```python
from build123d import *

# Parameters (mm, degrees)
SKETCH1_W                      = 116.84
SKETCH1_H                      = 76.2
EXTRUDE1_DEPTH                 = 6.35
F_1_4_CLEARANCE_HOLE1_D        = 6.7564
MIRROR2_COPY_1_D               = 6.7564
F_1_2_0_5_DIAMETER_HOLE1_D     = 12.7
F_1_2_0_5_DIAMETER_HOLE1_DEPTH = 17.78
F_1_2_0_5_DIAMETER_HOLE1_TIP   = 3.815464931


with BuildPart() as part:
    # Sketch1 → Extrude1 (new body)
    with BuildSketch(Plane.XY):
        Rectangle(SKETCH1_W, SKETCH1_H)
    extrude(amount=EXTRUDE1_DEPTH)

    # 1/4 Clearance Hole1 (through all)
    with Locations(Plane(origin=(-52.07, 31.75, 6.35), x_dir=(1, 0, 0), z_dir=(0, 0, 1))):
        with Locations((0, 0)):
            f_1_4_clearance_hole1 = Hole(F_1_4_CLEARANCE_HOLE1_D / 2)

    # Mirror1: 1/4 Clearance Hole1 across plane
    add(f_1_4_clearance_hole1.mirror(Plane.ZX), mode=Mode.SUBTRACT)

    # Mirror2: 1/4 Clearance Hole1 across plane
    add(f_1_4_clearance_hole1.mirror(Plane(origin=(0, 0, 0), x_dir=(0, 0, 1), z_dir=(1, 0, 0))), mode=Mode.SUBTRACT)

    # Mirror2 copy 1 (through all)
    with Locations(Plane(origin=(52.07, -31.75, 6.35), x_dir=(-1, 0, 0), z_dir=(0, 0, 1))):
        with Locations((0, 0)):
            Hole(MIRROR2_COPY_1_D / 2)

    # 1/2 (0.5) Diameter Hole1
    with Locations(Plane(origin=(-26.9875, 26.9875, 6.35), x_dir=(1, 0, 0), z_dir=(0, 0, 1))):
        with Locations((0, 0), (53.975, 0), (53.975, -53.975), (0, -53.975)):
            Hole(F_1_2_0_5_DIAMETER_HOLE1_D / 2, depth=F_1_2_0_5_DIAMETER_HOLE1_DEPTH)
            with Locations((0, 0, -(F_1_2_0_5_DIAMETER_HOLE1_DEPTH + F_1_2_0_5_DIAMETER_HOLE1_TIP / 2))):  # 118° drill point
                Cone(0, F_1_2_0_5_DIAMETER_HOLE1_D / 2, F_1_2_0_5_DIAMETER_HOLE1_TIP, mode=Mode.SUBTRACT)


solid = part.part
```
Can you work these out from the model? Positions are in its coordinate system, mm. Coordinates: 2 decimals unless noted, no trailing zeros. Loops run counter-clockwise (first coordinate to the right, second up) from the corner with the lowest first, then second, coordinate; pieces in that order, holes last.
Item 1: Suppose I cut it at C-C (z = 1). State how many separate pieces and enclosed holes the cut face has, then the cut area to 3 significant figures.
Answers below:
separate pieces: 1
enclosed holes: 8
area: 8,250 mm2
Item 2: Please list where these lines run through material, in increasing order: L1, parallel to Y at x = 52.07, z = 3.75; L2, parallel to Y at x = 29, z = 2; L3, parallel to X at y = -30, z = 1.
Answers below:
L1: y = -38.1 to -35.13, -28.37 to 28.37, 35.13 to 38.1
L2: y = -38.1 to -33.01, -20.96 to 20.96, 33.01 to 38.1
L3: x = -58.42 to -54.96, -49.18 to -32.58, -21.4 to 21.4, 32.58 to 49.18, 54.96 to 58.42
Item 3: Suppose I cut it at D-D (y = -30). Please give me the cut outline in (x, z), then the cut area to 3 significant figures.
Answers below:
outline: (-58.42, 0) - (-54.96, 0) - (-54.96, 6.35) - (-58.42, 6.35) - close; (-49.18, 0) - (-32.58, 0) - (-32.58, 6.35) - (-49.18, 6.35) - close; (-21.4, 0) - (21.4, 0) - (21.4, 6.35) - (-21.4, 6.35) - close; (32.58, 0) - (49.18, 0) - (49.18, 6.35) - (32.58, 6.35) - close; (54.96, 0) - (58.42, 0) - (58.42, 6.35) - (54.96, 6.35) - close
area: 527 mm2
Item 4: If we mould it in two halves opening along X, with no side actions, what happens to faces 1 (the face through (58.42, -1, 3)), 2 (the face through (-33.044, 28.895, 3.131)), 3 (the face through (-1, 1, 0))? For each: released by +X, released by -X, zero draft, split by the parting line, or undercut.
Answers below:
face 1: released by +X
face 2: undercut
face 3: zero draft
Item 5: Suppose I cut it at A-A (x = -52.07). Please give me the cut outline in (y, z), then the cut area to 3 significant figures.
Answers below:
outline: (-38.1, 0) - (-35.13, 0) - (-35.13, 6.35) - (-38.1, 6.35) - close; (-28.37, 0) - (28.37, 0) - (28.37, 6.35) - (-28.37, 6.35) - close; (35.13, 0) - (38.1, 0) - (38.1, 6.35) - (35.13, 6.35) - close
area: 398 mm2
Item 6: I'm going to push flat-ended pins straight in: pin 1 (7.5 mm diameter, centred on x = -26.99, y = 26.99, fed in from -Z); pin 2 (16.5 mm diameter, centred on x = 26.99, y = 26.99, fed in from -Z). Where does each tip first touch, or does it pass through?
Answers below:
pin 1: passes through
pin 2: stops at z = 0
Item 7: Suppose I cut it at B-B (y = 31.75). Please give me the cut outline in (x, z), then the cut area to 3 significant figures.
Answers below:
outline: (-58.42, 0) - (-55.45, 0) - (-55.45, 6.35) - (-58.42, 6.35) - close; (-48.69, 0) - (-31.19, 0) - (-31.19, 6.35) - (-48.69, 6.35) - close; (-22.79, 0) - (22.79, 0) - (22.79, 6.35) - (-22.79, 6.35) - close; (31.19, 0) - (48.69, 0) - (48.69, 6.35) - (31.19, 6.35) - close; (55.45, 0) - (58.42, 0) - (58.42, 6.35) - (55.45, 6.35) - close
area: 549 mm2
